Geometry: see drawing. Coordinates: mm, zero at the bounding-box minimum. Coordinates: 2 decimals unless noted, no trailing zeros. Loops run counter-clockwise (first coordinate to the right, second up) from the corner with the lowest first, then second, coordinate; pieces in that order, holes last. Notation, with made-up numbers: (49.25, 1.25) -> (93.25, 1.25) arc R35 cw to (93.25, 35.25) -> close; hole circle Ø9 at (-38.75, 49). An arc over 180 degrees is marked (long way). Answer as a JSON object with one key per item and string values.
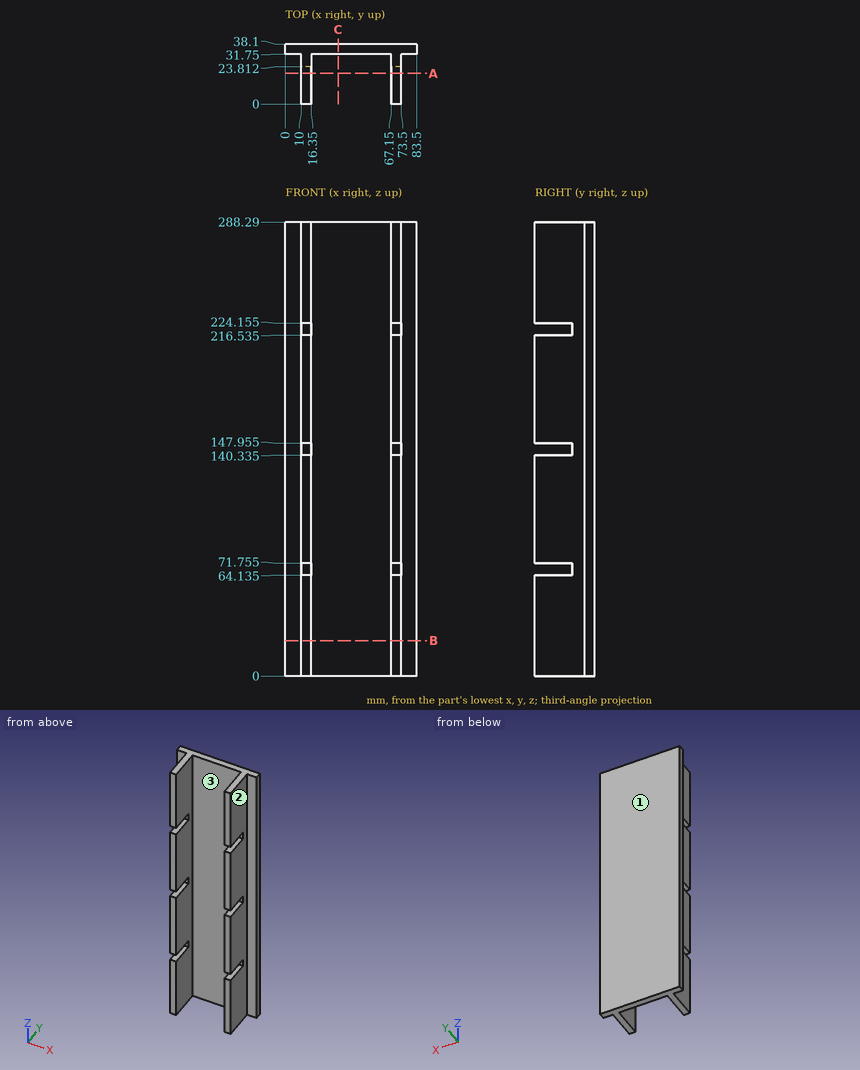
1. Pin query (flat end, axial travel): P1, Ø3, axis at x = 69.5, z = 144, coming from the -Y side; P2, Ø5, axis at x = 81, z = 143.5, coming from the -Y side; P3, Ø1.5, axis at y = 8.5, z = 117, coming from the -X side; P4, Ø6, axis at x = 21, y = 21.5, coming from the +Z side. Return the tip coordinate at first contact, or that it passes through.
Reply:
{"P1": "stops at y = 23.81", "P2": "stops at y = 31.75", "P3": "stops at x = 10", "P4": "passes through"}
2. Section query C-C (x = 33.5). Return loops of the section in (y, z), plus the area to 3 significant figures.
Reply:
{"outline": "(31.75, 0) -> (38.1, 0) -> (38.1, 288.29) -> (31.75, 288.29) -> close", "area": "1,830 mm2"}
3. Mould query, pull axis X, two halves, no side actions, for the marked faces 1, 2 and 3. Classes: pulls with the +X half, pulls with the -X half, needs draft (parallel to the pull), parting line crosses it, or undercut.
Reply:
{"face 1": "needs draft", "face 2": "pulls with the +X half", "face 3": "undercut"}
4. Line query: line 1 along Z through (x, y) = (72.5, 19) (1 decimal); line 2 along X through (y, z) = (11, 185); line 3 along Y through (x, z) = (56, 35). Output: solid intervals per line, ascending.
Reply:
{"line 1": "z = 0 to 64.1, 71.8 to 140.3, 148 to 216.5, 224.2 to 288.3", "line 2": "x = 10 to 16.35, 67.15 to 73.5", "line 3": "y = 31.75 to 38.1"}
5. Section query A-A (y = 19.5). Count the separate pieces of the cut face and the enclosed holes in it, plus the area to 3 significant figures.
Reply:
{"separate pieces": "8", "enclosed holes": "0", "area": "3,370 mm2"}
6. Section query B-B (z = 22.5). Return loops of the section in (x, y).
Reply:
{"outline": "(0, 31.75) -> (10, 31.75) -> (10, 0) -> (16.35, 0) -> (16.35, 31.75) -> (67.15, 31.75) -> (67.15, 0) -> (73.5, 0) -> (73.5, 31.75) -> (83.5, 31.75) -> (83.5, 38.1) -> (0, 38.1) -> close"}
